```python
from build123d import *

# Parameters (mm, degrees)
SKETCH2_W           = 50.8
SKETCH2_H           = 127
SKETCH2_R           = 14.351
SKETCH2_R_2         = 2.5527
BOSS_EXTRUDE3_DEPTH = 9.525
FILLET1_R           = 19.05
FILLET4_R           = 19.05


with BuildPart() as part:
    # Sketch2 → Boss-Extrude3 (new body)
    with BuildSketch(Plane.XY):
        with Locations((25.4, 63.5)):
            Rectangle(SKETCH2_W, SKETCH2_H)
        with Locations(Location((25.4, 96.5708, 0), (0, 0, 180))):
            Circle(SKETCH2_R, mode=Mode.SUBTRACT)
        with Locations(Location((43.1292, 114.3, 0), (0, 0, 180))):
            Circle(SKETCH2_R_2, mode=Mode.SUBTRACT)
        with Locations(Location((7.6708, 114.3, 0), (0, 0, 180))):
            Circle(SKETCH2_R_2, mode=Mode.SUBTRACT)
        with Locations(Location((7.6708, 78.8416, 0), (0, 0, 180))):
            Circle(SKETCH2_R_2, mode=Mode.SUBTRACT)
        with Locations(Location((43.1292, 78.8416, 0), (0, 0, 180))):
            Circle(SKETCH2_R_2, mode=Mode.SUBTRACT)
    extrude(amount=BOSS_EXTRUDE3_DEPTH)

    # Fillet1
    fillet1_edges = [part.edges().sort_by_distance(p)[0] for p in [
        (50.8, 127, 4.7625),
    ]]
    fillet(fillet1_edges, radius=FILLET1_R)

    # Fillet4
    fillet4_edges = [part.edges().sort_by_distance(p)[0] for p in [
        (0, 127, 4.7625),
    ]]
    fillet(fillet4_edges, radius=FILLET4_R)


solid = part.part
```
Geometry check sheet. Reference: the model listing, model coordinates, mm. Coordinates: 2 decimals unless noted, no trailing zeros. Write each loop counter-clockwise with the first axis right and the second up, starting at its lowest first coordinate (ties: lowest second). Pieces come first, ordered by that corner, then holes. Notation, with made-up numbers: (13.5, 26) -> (18.5, 26) arc R28 ccw to (18.5, 52) -> close; hole circle Ø11 at (85.25, -19). An arc over 180 degrees is marked (long way). Use CSV: the item, a comma, the result in double quotes. Start each with the question number.
Item 1: Thickness scan on line 1 (X direction, y = 114.3, z = 2.25); line 2 (Y direction, x = 25.4, z = 3.75); line 3 (Y direction, x = 45, z = 2.25). Record the ranges inside material, lowest first.
Item 2: Cross-section at D-D, the plane x = 4. Record the cut outline in (y, z) (3 decimals), plus the area to 3 significant figures.
Item 3: Mould release check, pull along X, two halves, no side actions. Record for faces 1 (the cylindrical face through (27.268, 82.342, 4.696)), 2 (the flat face through (25, 64, 9.525)), 3 (the cylindrical face through (43.683, 81.334, 4.696)), 4 (the cylindrical face through (5.73, 121.57, 4.83)): released by +X, released by -X, zero draft, split by the parting line, or undercut.
Item 4: Cross-section at B-B, the plane y = 114.3. Record the cut outline in (x, z) (1 decimal).
Item 5: Cross-section at A-A, the plane x = 25.4. Record the cut outline in (y, z) (3 decimals), plus the area to 3 significant figures.
Item 6: Cross-section at C-C, the plane z = 6.5. Record the cut outline in (x, y), plus the area to 3 significant figures.
Answers:
1,line 1,"1.09 to 5.12, 10.22 to 40.58, 45.68 to 49.71"
1,line 2,"0 to 82.22, 110.92 to 127"
1,line 3,"0 to 77.1, 80.58 to 112.56, 116.04 to 121.64"
2,outline,"(0, 0) -> (119.629, 0) -> (119.629, 9.525) -> (0, 9.525) -> close"
2,area,"1,140 mm^2"
3,face 1,"undercut"
3,face 2,"zero draft"
3,face 3,"undercut"
3,face 4,"released by -X"
4,outline,"(1.1, 0) -> (5.1, 0) -> (5.1, 9.5) -> (1.1, 9.5) -> close; (10.2, 0) -> (40.6, 0) -> (40.6, 9.5) -> (10.2, 9.5) -> close; (45.7, 0) -> (49.7, 0) -> (49.7, 9.5) -> (45.7, 9.5) -> close"
5,outline,"(0, 0) -> (82.22, 0) -> (82.22, 9.525) -> (0, 9.525) -> close; (110.922, 0) -> (127, 0) -> (127, 9.525) -> (110.922, 9.525) -> close"
5,area,"936 mm^2"
6,outline,"(0, 0) -> (50.8, 0) -> (50.8, 107.95) arc R19.05 ccw to (31.75, 127) -> (19.05, 127) arc R19.05 ccw to (0, 107.95) -> close; hole circle Ø5.11 at (7.67, 78.84); hole circle Ø5.11 at (7.67, 114.3); hole circle Ø28.7 at (25.4, 96.57); hole circle Ø5.11 at (43.13, 78.84); hole circle Ø5.11 at (43.13, 114.3)"
6,area,"5,570 mm^2"
